```python
from build123d import *


with BuildPart() as f2:
    # F2: sweep along a path in F1
    with BuildLine(Plane.YZ) as f2_path:
        Line((0, 0), (235.4986518621, 0))
        Line((235.4986518621, 0), (235.4986518621, 181.7011833191))
        Line((235.4986518621, 181.7011833191), (405.3635597229, 181.7011833191))
        Line((405.3635597229, 181.7011833191), (410.0448787212, -205.5106014013))
    # F0 (on Front) → F2 (sweep)
    with BuildSketch(Plane.XZ):
        with BuildLine():
            Line((-43.4998961684, 38.1), (-43.4998961684, -38.1))
            ThreePointArc((-43.4998961684, -38.1), (-39.7801522895, -47.0802561211), (-30.7998961684, -50.8))
            Line((-30.7998961684, -50.8), (45.4001038316, -50.8))
            ThreePointArc((45.4001038316, -50.8), (54.3803599527, -47.0802561211), (58.1001038316, -38.1))
            Line((58.1001038316, -38.1), (58.1001038316, 38.1))
            ThreePointArc((58.1001038316, 38.1), (54.3803599527, 47.0802561211), (45.4001038316, 50.8))
            Line((45.4001038316, 50.8), (-30.7998961684, 50.8))
            ThreePointArc((-30.7998961684, 50.8), (-39.7801522895, 47.0802561211), (-43.4998961684, 38.1))
        make_face()
        with BuildLine():
            ThreePointArc((-37.1498961684, 31.75), (-33.4301522895, 40.7302561211), (-24.4498961684, 44.45))
            Line((-24.4498961684, 44.45), (39.0501038316, 44.45))
            ThreePointArc((39.0501038316, 44.45), (48.0303599527, 40.7302561211), (51.7501038316, 31.75))
            Line((51.7501038316, 31.75), (51.7501038316, -31.75))
            ThreePointArc((51.7501038316, -31.75), (48.0303599527, -40.7302561211), (39.0501038316, -44.45))
            Line((39.0501038316, -44.45), (-24.4498961684, -44.45))
            ThreePointArc((-24.4498961684, -44.45), (-33.4301522895, -40.7302561211), (-37.1498961684, -31.75))
            Line((-37.1498961684, -31.75), (-37.1498961684, 31.75))
        make_face(mode=Mode.SUBTRACT)
    sweep(path=f2_path.line, transition=Transition.RIGHT)


solid = f2.part
```
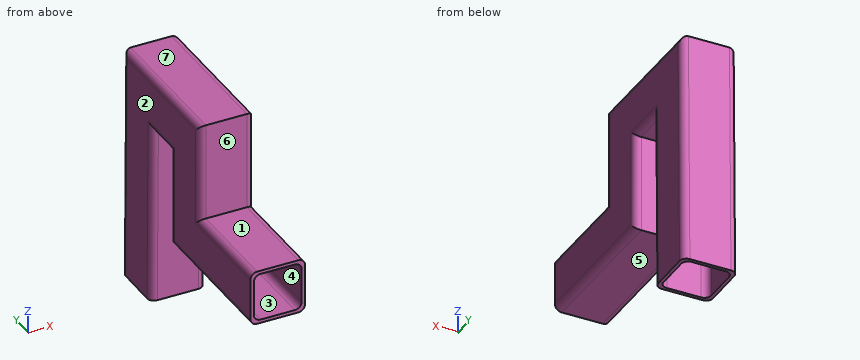
The listing builds one solid part. Answer for the finished solid, in the listing's coordinates (mm). Face numbers are marked on the shaded views. A direction names the side the tool comes from. Round coordinates to 2 decimals unless told otherwise and drop trailing zeros. Order: outer loops, then holes, each group sorted by start corner. A loop starts at its lowest first (then second) coordinate and runs counter-clockwise, first axis right, second up. Notation, with made-up numbers: (44, 60) -> (99, 60) arc R22 ccw to (99, 68) -> close; hole circle Ø2 at (-13, 41.5). An arc over 180 degrees is marked (long way). Answer as CSV lines item,"result". Start each with the question number.
(1) For a pull along Z with two mould halves and no side action, classify the marked faces 1, 2 and 3 as +Z half, -Z half, draft (parallel to the pull), parting line (faces both ways), or undercut.
(2) Find the intervals of material crossed by probe 1 along Z at (x, y) = (0.5, 51); probe 2 along Y at (x, z) = (-20.5, 37); probe 3 along Z at (x, y) = (-3.5, 186), in increasing order. Write a range as from..to.
(3) The part is cut by section D-D (y = 407). Determine the outline of the cut face in (x, z).
(4) The part is cut by section A-A (x = 10). Determine the outline of the cut face in (y, z).
(5) Flat-ended cylindrical pins translate along their axes: pin 1 Ø19 at (x, z) = (7, 85.5) entering from -Y; pin 2 Ø5 at (x, y) = (25.5, 208) entering from -Z; pin 3 Ø19 at (x, y) = (18, 375.5) entering from -Z. Find the tip coordinate at first contact, or state that the pin passes through.
(6) The part is cut by section B-B (y = 97). Determine the outline of the cut face in (x, z).
(7) A tool of negligible diameter and unlimited length cuts with its end or side. For the marked faces 4, 5, 6 and 7, from which of +Z, -Z, +X, -X, +Y, -Y can it reach the whole face along a straight path? Write none if from no direction.
(8) The part is cut by section C-C (z = 22). Count the separate pieces of the cut face and the enclosed holes in it, then the cut area to 3 significant figures.
Evaluation:
1,face 1,"+Z half"
1,face 2,"draft"
1,face 3,"undercut"
2,probe 1,"-50.8..-44.45, 44.45..50.8"
2,probe 2,"279.95..286.3, 356.31..362.66, 451.57..457.92"
2,probe 3,"-50.8..-44.45, 44.45..232.5"
3,outline,"(-43.5, -205.55) -> (-37.15, -205.55) -> (-37.15, 213.45) arc R12.7 cw to (-24.45, 226.15) -> (39.05, 226.15) arc R12.7 cw to (51.75, 213.45) -> (51.75, -205.55) -> (58.1, -205.55) -> (58.1, 219.8) arc R12.7 ccw to (45.4, 232.5) -> (-30.8, 232.5) arc R12.7 ccw to (-43.5, 219.8) -> close"
4,outline,"(0, -50.8) -> (286.3, -50.8) -> (286.3, 130.9) -> (355.17, 130.9) -> (359.25, -206.12) -> (365.6, -206.05) -> (361.45, 137.25) -> (279.95, 137.25) -> (279.95, -44.45) -> (0, -44.45) -> close; (0, 44.45) -> (191.05, 44.45) -> (191.05, 226.15) -> (449.28, 226.15) -> (454.49, -204.97) -> (460.84, -204.9) -> (455.55, 232.5) -> (184.7, 232.5) -> (184.7, 50.8) -> (0, 50.8) -> close"
5,pin 1,"y = 184.7"
5,pin 2,"z = -50.8"
5,pin 3,"z = 226.15"
6,outline,"(-43.5, -38.1) arc R12.7 ccw to (-30.8, -50.8) -> (45.4, -50.8) arc R12.7 ccw to (58.1, -38.1) -> (58.1, 38.1) arc R12.7 ccw to (45.4, 50.8) -> (-30.8, 50.8) arc R12.7 ccw to (-43.5, 38.1) -> close; hole (-37.15, -31.75) arc R12.7 ccw to (-24.45, -44.45) -> (39.05, -44.45) arc R12.7 ccw to (51.75, -31.75) -> (51.75, 31.75) arc R12.7 ccw to (39.05, 44.45) -> (-24.45, 44.45) arc R12.7 ccw to (-37.15, 31.75) -> close"
7,face 4,"none"
7,face 5,"-Z, +X, -X, -Y"
7,face 6,"+Z, +X, -X, -Y"
7,face 7,"+Z, +X, -X, +Y, -Y"
8,separate pieces,"2"
8,enclosed holes,"1"
8,area,"6,620 mm²"
